Geometry check sheet. Reference: the model listing, model coordinates, mm. Give positions to 0.01 mm unless a question says otherwise; leave off trailing zeros. Loops run counter-clockwise (first coordinate to the right, second up) from the corner with the lowest first, then second, coordinate; pieces in that order, holes last.
```python
from build123d import *

# Parameters (mm, degrees)
SKETCH4_W                   = 177.8
SKETCH4_H                   = 76.2
BOSS_EXTRUDE3_DEPTH         = 1.5
SOLENOID_PANEL_CUTOUTS_R    = 1.55
SOLENOID_PANEL_CUTOUTS_W    = 11.8
SOLENOID_PANEL_CUTOUTS_H    = 18.7
SOLENOID_PANEL_CUTOUT_DEPTH = 1.5


with BuildPart() as part:
    # Sketch4 → Boss-Extrude3 (new body)
    with BuildSketch(Plane(origin=(0, 0, 0), x_dir=(1, 0, 0), z_dir=(0, 1, 0))):
        with Locations((88.9, 38.1)):
            Rectangle(SKETCH4_W, SKETCH4_H)
    extrude(amount=BOSS_EXTRUDE3_DEPTH)

    # Solenoid Panel Cutouts → Solenoid Panel Cutout (cut)
    with BuildSketch(Plane(origin=(0, 0, 0), x_dir=(1, 0, 0), z_dir=(0, 1, 0))):
        with Locations(Location((10.743745769, 33.162501773, 0), (0, 0, 90))):
            Circle(SOLENOID_PANEL_CUTOUTS_R)
        with Locations(Location((10.743745769, 4.937501773, 0), (0, 0, 90))):
            Circle(SOLENOID_PANEL_CUTOUTS_R)
        with Locations(Location((10.743745769, 71.262501773, 0), (0, 0, 90))):
            Circle(SOLENOID_PANEL_CUTOUTS_R)
        with Locations(Location((10.743745769, 43.037501773, 0), (0, 0, 90))):
            Circle(SOLENOID_PANEL_CUTOUTS_R)
        with Locations(Location((47.256245769, 71.262501773, 0), (0, 0, 90))):
            Circle(SOLENOID_PANEL_CUTOUTS_R)
        with Locations(Location((47.256245769, 43.037501773, 0), (0, 0, 90))):
            Circle(SOLENOID_PANEL_CUTOUTS_R)
        with Locations(Location((70.643745769, 71.262501773, 0), (0, 0, 90))):
            Circle(SOLENOID_PANEL_CUTOUTS_R)
        with Locations(Location((70.643745769, 43.037501773, 0), (0, 0, 90))):
            Circle(SOLENOID_PANEL_CUTOUTS_R)
        with Locations(Location((107.156245769, 71.262501773, 0), (0, 0, 90))):
            Circle(SOLENOID_PANEL_CUTOUTS_R)
        with Locations(Location((107.156245769, 43.037501773, 0), (0, 0, 90))):
            Circle(SOLENOID_PANEL_CUTOUTS_R)
        with Locations(Location((130.543745769, 71.262501773, 0), (0, 0, 90))):
            Circle(SOLENOID_PANEL_CUTOUTS_R)
        with Locations(Location((130.543745769, 43.037501773, 0), (0, 0, 90))):
            Circle(SOLENOID_PANEL_CUTOUTS_R)
        with Locations(Location((167.056245769, 71.262501773, 0), (0, 0, 90))):
            Circle(SOLENOID_PANEL_CUTOUTS_R)
        with Locations(Location((167.056245769, 43.037501773, 0), (0, 0, 90))):
            Circle(SOLENOID_PANEL_CUTOUTS_R)
        with Locations(Location((28.999995769, 52.212501773, 0), (0, 0, 90))):
            Circle(SOLENOID_PANEL_CUTOUTS_R)
        with Locations(Location((28.999995769, 23.987501773, 0), (0, 0, 90))):
            Circle(SOLENOID_PANEL_CUTOUTS_R)
        with Locations(Location((47.256245769, 33.162501773, 0), (0, 0, 90))):
            Circle(SOLENOID_PANEL_CUTOUTS_R)
        with Locations(Location((47.256245769, 4.937501773, 0), (0, 0, 90))):
            Circle(SOLENOID_PANEL_CUTOUTS_R)
        with Locations(Location((70.643745769, 33.162501773, 0), (0, 0, 90))):
            Circle(SOLENOID_PANEL_CUTOUTS_R)
        with Locations(Location((70.643745769, 4.937501773, 0), (0, 0, 90))):
            Circle(SOLENOID_PANEL_CUTOUTS_R)
        with Locations(Location((88.899995769, 52.212501773, 0), (0, 0, 90))):
            Circle(SOLENOID_PANEL_CUTOUTS_R)
        with Locations(Location((88.899995769, 23.987501773, 0), (0, 0, 90))):
            Circle(SOLENOID_PANEL_CUTOUTS_R)
        with Locations(Location((107.156245769, 33.162501773, 0), (0, 0, 90))):
            Circle(SOLENOID_PANEL_CUTOUTS_R)
        with Locations(Location((107.156245769, 4.937501773, 0), (0, 0, 90))):
            Circle(SOLENOID_PANEL_CUTOUTS_R)
        with Locations(Location((130.543745769, 33.162501773, 0), (0, 0, 90))):
            Circle(SOLENOID_PANEL_CUTOUTS_R)
        with Locations(Location((130.543745769, 4.937501773, 0), (0, 0, 90))):
            Circle(SOLENOID_PANEL_CUTOUTS_R)
        with Locations(Location((148.799995769, 52.212501773, 0), (0, 0, 90))):
            Circle(SOLENOID_PANEL_CUTOUTS_R)
        with Locations(Location((148.799995769, 23.987501773, 0), (0, 0, 90))):
            Circle(SOLENOID_PANEL_CUTOUTS_R)
        with Locations(Location((167.056245769, 33.162501773, 0), (0, 0, 90))):
            Circle(SOLENOID_PANEL_CUTOUTS_R)
        with Locations(Location((167.056245769, 4.937501773, 0), (0, 0, 90))):
            Circle(SOLENOID_PANEL_CUTOUTS_R)
        with Locations((10.743745769, 19.050001773)):
            Rectangle(SOLENOID_PANEL_CUTOUTS_W, SOLENOID_PANEL_CUTOUTS_H)
        with Locations((10.743745769, 57.150001773)):
            Rectangle(SOLENOID_PANEL_CUTOUTS_W, SOLENOID_PANEL_CUTOUTS_H)
        with Locations((47.256245769, 57.150001773)):
            Rectangle(SOLENOID_PANEL_CUTOUTS_W, SOLENOID_PANEL_CUTOUTS_H)
        with Locations((70.643745769, 57.150001773)):
            Rectangle(SOLENOID_PANEL_CUTOUTS_W, SOLENOID_PANEL_CUTOUTS_H)
        with Locations((107.156245769, 57.150001773)):
            Rectangle(SOLENOID_PANEL_CUTOUTS_W, SOLENOID_PANEL_CUTOUTS_H)
        with Locations((130.543745769, 57.150001773)):
            Rectangle(SOLENOID_PANEL_CUTOUTS_W, SOLENOID_PANEL_CUTOUTS_H)
        with Locations((167.056245769, 57.150001773)):
            Rectangle(SOLENOID_PANEL_CUTOUTS_W, SOLENOID_PANEL_CUTOUTS_H)
        with Locations((28.999995769, 38.100001773)):
            Rectangle(SOLENOID_PANEL_CUTOUTS_W, SOLENOID_PANEL_CUTOUTS_H)
        with Locations((47.256245769, 19.050001773)):
            Rectangle(SOLENOID_PANEL_CUTOUTS_W, SOLENOID_PANEL_CUTOUTS_H)
        with Locations((70.643745769, 19.050001773)):
            Rectangle(SOLENOID_PANEL_CUTOUTS_W, SOLENOID_PANEL_CUTOUTS_H)
        with Locations((88.899995769, 38.100001773)):
            Rectangle(SOLENOID_PANEL_CUTOUTS_W, SOLENOID_PANEL_CUTOUTS_H)
        with Locations((107.156245769, 19.050001773)):
            Rectangle(SOLENOID_PANEL_CUTOUTS_W, SOLENOID_PANEL_CUTOUTS_H)
        with Locations((130.543745769, 19.050001773)):
            Rectangle(SOLENOID_PANEL_CUTOUTS_W, SOLENOID_PANEL_CUTOUTS_H)
        with Locations((148.799995769, 38.100001773)):
            Rectangle(SOLENOID_PANEL_CUTOUTS_W, SOLENOID_PANEL_CUTOUTS_H)
        with Locations((167.056245769, 19.050001773)):
            Rectangle(SOLENOID_PANEL_CUTOUTS_W, SOLENOID_PANEL_CUTOUTS_H)
    extrude(amount=SOLENOID_PANEL_CUTOUT_DEPTH, mode=Mode.SUBTRACT)


solid = part.part
```
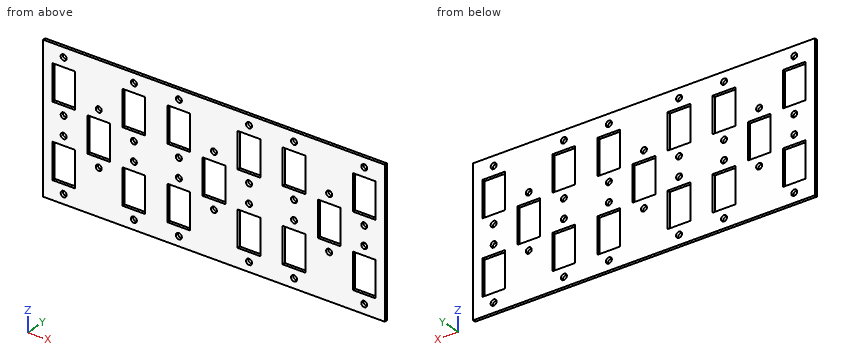
1) Sectioned sample at C-C on y = 0.95. Count the separate pieces of the cut face and the enclosed holes in it, plus the area to 3 significant figures.
2) Sectioned sample at A-A on z = -17. Enter the section's corners in (x, y).
3) Sectioned sample at B-B on x = 51.5. Enter the section's corners in (y, z).
4) Scan lines: line 1 along Z through (x, y) = (29, 0.8); line 2 along X through (y, z) = (1.4, -40); line 3 along Z through (x, y) = (170, 0.45). Record each from-to range of solid material in increasing order.
Determined:
1. separate pieces: 1
1. enclosed holes: 45
1. area: 10,000 mm2
2. outline: (0, 0) - (4.84, 0) - (4.84, 1.5) - (0, 1.5) - close; (16.64, 0) - (41.36, 0) - (41.36, 1.5) - (16.64, 1.5) - close; (53.16, 0) - (64.74, 0) - (64.74, 1.5) - (53.16, 1.5) - close; (76.54, 0) - (101.26, 0) - (101.26, 1.5) - (76.54, 1.5) - close; (113.06, 0) - (124.64, 0) - (124.64, 1.5) - (113.06, 1.5) - close; (136.44, 0) - (161.16, 0) - (161.16, 1.5) - (136.44, 1.5) - close; (172.96, 0) - (177.8, 0) - (177.8, 1.5) - (172.96, 1.5) - close
3. outline: (0, -76.2) - (1.5, -76.2) - (1.5, -66.5) - (0, -66.5) - close; (0, -47.8) - (1.5, -47.8) - (1.5, -28.4) - (0, -28.4) - close; (0, -9.7) - (1.5, -9.7) - (1.5, 0) - (0, 0) - close
4. line 1: z = -76.2 to -53.76, -50.66 to -47.45, -28.75 to -25.54, -22.44 to 0
4. line 2: x = 0 to 23.1, 34.9 to 83, 94.8 to 142.9, 154.7 to 177.8
4. line 3: z = -76.2 to -66.5, -47.8 to -28.4, -9.7 to 0
